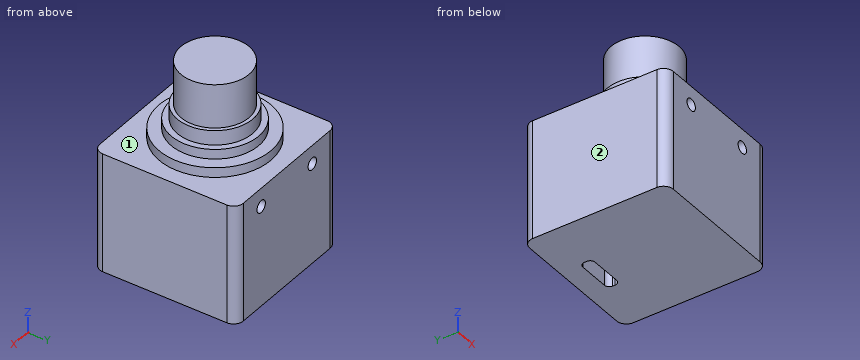
Autodesk Inventor part; units mm, degrees
ref_plane "YZ Plane" through (0, 0, 0) normal (1, 0, 0) x (0, 1, 0)
ref_plane "XZ Plane" through (0, 0, 0) normal (0, 1, 0) x (-1, 0, 0)
ref_plane "XY Plane" through (0, 0, 0) normal (0, 0, 1) x (1, 0, 0)
sketch "Sketch1" plane through (0, 0, 0) normal (0, 0, 1) x (1, 0, 0)
  line L0 (-14.75, 14.75) -> (14.75, 14.75)
  line L1 (14.75, 14.75) -> (14.75, -14.75)
  line L2 (14.75, -14.75) -> (-14.75, -14.75)
  line L3 (-14.75, -14.75) -> (-14.75, 14.75)
  line L4 (0, 0) -> (0, 4.6825) construction
  line L5 (0, 0) -> (4.0135, 0) construction
  dimension "d0" = 29.5
  dimension "d1" = 29.5
extrude "Extrusion1" add sketch "Sketch1" along normal blind 24.5
sketch "Sketch2" plane through (0, 0, 24.5) normal (0, 0, 1) x (1, 0, 0)
  circle A0 centre (0, 0) radius 11.5
  dimension "d4" = 23
extrude "Extrusion2" add sketch "Sketch2" along normal blind 2
sketch "Sketch3" plane through (0, 0, 26.5) normal (0, 0, 1) x (1, 0, 0)
  circle A0 centre (0, 0) radius 9
  dimension "d7" = 18
extrude "Extrusion3" add sketch "Sketch3" along normal blind 2
sketch "Sketch4" plane through (0, 0, 28.5) normal (0, 0, 1) x (1, 0, 0)
  circle A0 centre (0, 0) radius 7.75
  dimension "d10" = 15.5
extrude "Extrusion4" add sketch "Sketch4" along normal blind 3
sketch "Sketch5" plane through (0, 0, 31.5) normal (0, 0, 1) x (1, 0, 0)
  circle A0 centre (0, 0) radius 7
  dimension "d13" = 14
extrude "Extrusion5" add sketch "Sketch5" along normal blind 9
sketch "Sketch6" plane through (-14.75, 14.75, 0) normal (0, 1, 0) x (1, 0, 0)
  line L0 (29.5, -24.5) -> (0, -24.5)
  line L1 (0, 0) -> (0, -24.5)
  point P0 (14.75, 0)
  point P1 (7.25, -20.7)
  point P2 (22.25, -20.7)
  dimension "d16" = 15
  dimension "d17" = 3.8
  dimension "d18" = 7.25
hole "Hole1" at (-7.5, 14.75, 20.7) at (7.5, 14.75, 20.7) direction (0, -1, 0) diameter 2.459 depth 3 tip angle 118
fillet "Fillet1" radius 2 4 edges at (14.75, 14.75, 12.25) (-14.75, 14.75, 12.25) (-14.75, -14.75, 12.25) (14.75, -14.75, 12.25)
sketch "Sketch7" plane through (-12.75, -14.75, 0) normal (0, -1, 0) x (1, 0, 0)
  line L0 (0, 24.5) -> (25.5, 24.5)
  line L1 (-2, 24.5) -> (-2, 0)
  point P0 (12.75, 0)
  point P1 (5.25, 20.7)
  point P2 (20.25, 20.7)
  dimension "d27" = 15
  dimension "d28" = 3.8
  dimension "d29" = 7.25
hole "Hole2" at (-7.5, -14.75, 20.7) at (7.5, -14.75, 20.7) direction (0, 1, 0) diameter 2.459 depth 3 tip angle 118
sketch "Sketch8" plane through (0, 0, 0) normal (0, 0, -1) x (-1, 0, 0)
  line L0 (5.0435, 9.3) -> (-5.0435, 9.3) construction
  line L1 (3.15, 10.55) -> (-3.15, 10.55)
  line L2 (-3.15, 8.05) -> (3.15, 8.05)
  line L3 (0, 0) -> (-20.3594, 0) construction
  line L4 (0, 0) -> (0, -6.0077) construction
  line L5 (4.15, 9.05) -> (4.15, 9.55)
  line L6 (-4.15, 9.05) -> (-4.15, 9.55)
  arc A0 (3.15, 8.05) -> (4.15, 9.05) centre (3.15, 9.05) ccw
  arc A1 (4.15, 9.55) -> (3.15, 10.55) centre (3.15, 9.55) ccw
  arc A2 (-3.15, 10.55) -> (-4.15, 9.55) centre (-3.15, 9.55) ccw
  arc A3 (-4.15, 9.05) -> (-3.15, 8.05) centre (-3.15, 9.05) ccw
  point P0 (-4.15, 8.05)
  point P1 (4.15, 8.05)
  point P2 (0, 9.3)
  point P3 (-4.15, 10.55)
  dimension "d37" = 9.3
  dimension "d38" = 8.3
  dimension "d39" = 2.5
  dimension "d41" = 1
extrude "Extrusion6" cut sketch "Sketch8" against normal blind 6.5
properties part number "3d_JacintoDevKit_Addon - Camera"
Verification items for the finished model (mm, model axes). Face numbers are marked on the shaded views. A direction names the side the tool comes from. Give positions to 0.01 mm unless a question says otherwise; leave off trailing zeros. Order: outer loops, then holes, each group sorted by start corner. A loop starts at its lowest first (then second) coordinate and runs counter-clockwise, first axis right, second up. Notation, with made-up numbers: (85.25, 40) - (124.25, 40) arc R21 cw to (124.25, 76) - close; hole circle Ø6 at (9.5, -33). An arc over 180 degrees is marked (long way). Answer as CSV lines item,"result". Start each with the question number.
Item 1: Section check B-B, the plane x = 0. Record the boundary of the cut face in (y, z), plus the area to 3 significant figures.
Item 2: Section check C-C, the plane z = 34.5. Record the boundary of the cut face in (x, y), plus the area to 3 significant figures.
Item 3: Section check A-A, the plane y = 0. Record the boundary of the cut face in (x, z).
Item 4: Gauge pin test, flat ends, axial feed: pin 1 (1.5 mm diameter, centred on x = 7.5, z = 20.7, fed in from +Y); pin 2 (2 mm diameter, centred on x = 0.5, y = 9.5, fed in from -Z). Record the tip position at first contact, or that the pin passes through.
Item 5: Section check D-D, the plane y = 3.5. Record the boundary of the cut face in (x, z).
Item 6: Access from +Z, -Z, +X, -X, +Y, -Y to the whole of each face (thin tool, end or side, straight path). Record for the marked faces 1 and 2.
Item 7: Material ranges on L1, parallel to X at y = 12.7, z = 20.7; L2, parallel to Z at x = -7.5, y = -13.95; L3, parallel to X at y = -13.5, z = 20.7, recorded low to high.
Filled in:
1,outline,"(-14.75, 0) - (8.05, 0) - (8.05, 6.5) - (10.55, 6.5) - (10.55, 0) - (14.75, 0) - (14.75, 24.5) - (11.5, 24.5) - (11.5, 26.5) - (9, 26.5) - (9, 28.5) - (7.75, 28.5) - (7.75, 31.5) - (7, 31.5) - (7, 40.5) - (-7, 40.5) - (-7, 31.5) - (-7.75, 31.5) - (-7.75, 28.5) - (-9, 28.5) - (-9, 26.5) - (-11.5, 26.5) - (-11.5, 24.5) - (-14.75, 24.5) - close"
1,area,"961 mm^2"
2,outline,"circle Ø14 at (0, 0)"
2,area,"154 mm^2"
3,outline,"(-14.75, 0) - (14.75, 0) - (14.75, 24.5) - (11.5, 24.5) - (11.5, 26.5) - (9, 26.5) - (9, 28.5) - (7.75, 28.5) - (7.75, 31.5) - (7, 31.5) - (7, 40.5) - (-7, 40.5) - (-7, 31.5) - (-7.75, 31.5) - (-7.75, 28.5) - (-9, 28.5) - (-9, 26.5) - (-11.5, 26.5) - (-11.5, 24.5) - (-14.75, 24.5) - close"
4,pin 1,"y = 11.46"
4,pin 2,"z = 6.5"
5,outline,"(-14.75, 0) - (14.75, 0) - (14.75, 24.5) - (10.95, 24.5) - (10.95, 26.5) - (8.29, 26.5) - (8.29, 28.5) - (6.91, 28.5) - (6.91, 31.5) - (6.06, 31.5) - (6.06, 40.5) - (-6.06, 40.5) - (-6.06, 31.5) - (-6.91, 31.5) - (-6.91, 28.5) - (-8.29, 28.5) - (-8.29, 26.5) - (-10.95, 26.5) - (-10.95, 24.5) - (-14.75, 24.5) - close"
6,face 1,"+Z"
6,face 2,"+Z, -Z, -X, +Y, -Y"
7,L1,"-14.75 to -8.73, -6.27 to 6.27, 8.73 to 14.75"
7,L2,"0 to 19.47, 21.93 to 24.5"
7,L3,"-14.6 to -8.73, -6.27 to 6.27, 8.73 to 14.6"
